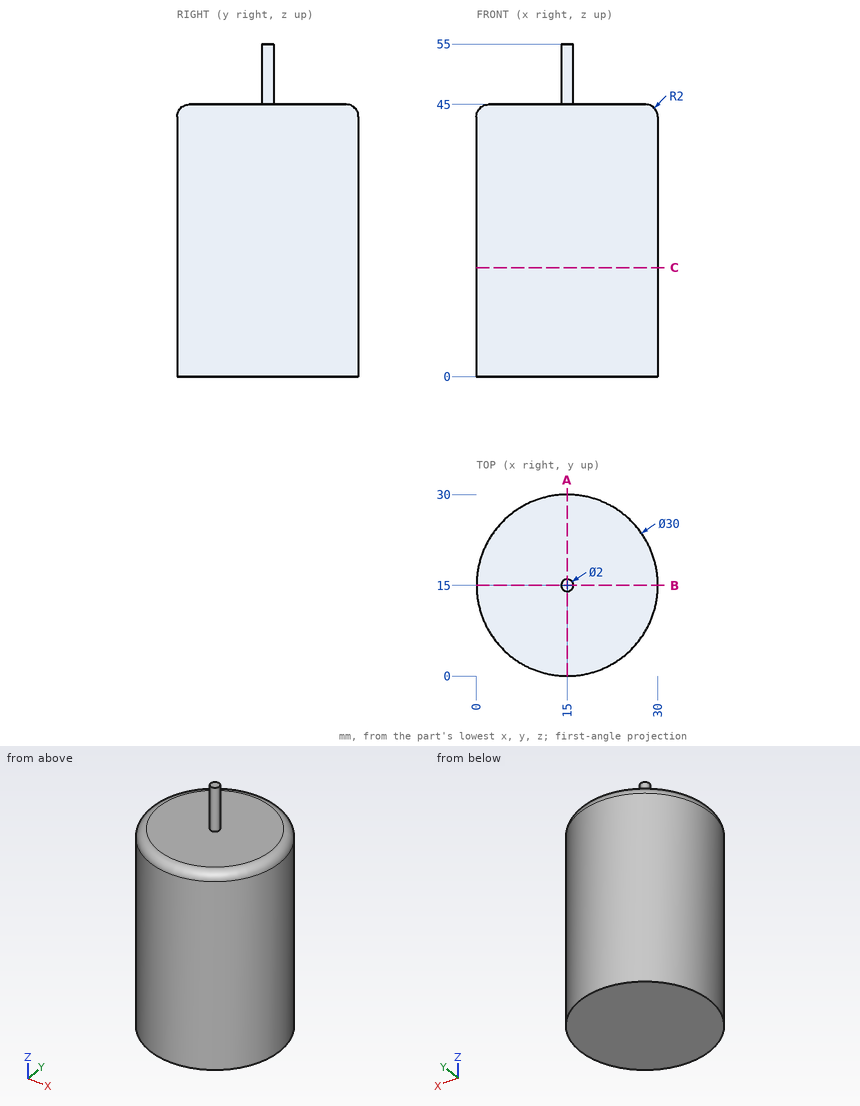
Part print with two shaded views. Sizes in mm from the minimum x, y, z corner. Coordinates: 2 decimals unless noted, no trailing zeros. Write each loop counter-clockwise with the first axis right and the second up, starting at its lowest first coordinate (ties: lowest second). Pieces come first, ordered by that corner, then holes.
(1) Cut at A-A on x = 15. List the corners of the cut face in (y, z), and give its area (3 significant figures).
(2) Drill centre lines: line 1 (Z direction, x = 5, y = 19.25); line 2 (Y direction, x = 21, z = 27.5). Where is each one in solid material? Low to high.
(3) Pin check, flat tips, straight feed: pin 1 Ø5 at (y, z) = (10.5, 42.5) entering from -X; pin 2 Ø4 at (x, y) = (11.5, 21.5) entering from -Z; pin 3 Ø1 at (y, z) = (5.5, 19) entering from -X; pin 4 Ø1.5 at (y, z) = (3.5, 46.5) entering from -X. Stop position of each tip, or through.
(4) Cut at C-C on z = 18. List the corners of the cut face in (x, y).
Working result:
1. outline: (0, 0) - (30, 0) - (30, 43) arc R2 ccw to (28, 45) - (16, 45) - (16, 55) - (14, 55) - (14, 45) - (2, 45) arc R2 ccw to (0, 43) - close
1. area: 1,370 mm2
2. line 1: z = 0 to 45
2. line 2: y = 1.25 to 28.75
3. pin 1: stops at x = 0.13
3. pin 2: stops at z = 0
3. pin 3: stops at x = 3
3. pin 4: passes through
4. outline: circle Ø30 at (15, 15)
